Geometry: final body of the model. Coordinates: model frame, mm. A direction names the side the tool comes from. Coordinates: 2 decimals unless noted, no trailing zeros. Loops run counter-clockwise (first coordinate to the right, second up) from the corner with the lowest first, then second, coordinate; pieces in that order, holes last. Notation, with made-up numbers: (53, 41) - (59, 41) arc R13 ccw to (59, 59) - close; hole circle Ø7 at (-5, 17). An arc over 180 degrees is marked (long way). Return JSON: item names as keys, results as strings.
from build123d import *

# Parameters (mm, degrees)
SKETCH1_R           = 1
BOSS_EXTRUDE1_DEPTH = 4
SKETCH2_R           = 1
CUT_EXTRUDE1_DEPTH  = 4


with BuildPart() as part:
    # Sketch1 → Boss-Extrude1 (new body)
    with BuildSketch(Plane(origin=(0, 0, 0), x_dir=(1, 0, 0), z_dir=(0, 1, 0))):
        Polygon((0, 0), (47.5, 0), (72.5, 25), (72.5, 50), (62.5, 50), (62.5, 29.142135624), (43.357864376, 10), (0, 10), (-43.357864376, 10), (-62.5, 29.142135624), (-62.5, 50), (-72.5, 50), (-72.5, 25), (-47.5, 0), align=None)
        with Locations(Location((10, 5, 0), (0, 0, 270))):
            Circle(SKETCH1_R, mode=Mode.SUBTRACT)
        with Locations(Location((0, 5, 0), (0, 0, 270))):
            Circle(SKETCH1_R, mode=Mode.SUBTRACT)
        with Locations(Location((-10, 5, 0), (0, 0, 90))):
            Circle(SKETCH1_R, mode=Mode.SUBTRACT)
    extrude(amount=BOSS_EXTRUDE1_DEPTH)

    # Sketch2 → Cut-Extrude1 (cut)
    with BuildSketch(Plane(origin=(0, 4, 0), x_dir=(1, 0, 0), z_dir=(0, 1, 0))):
        with Locations(Location((67.5, 47.5, 0), (0, 0, 270))):
            Circle(SKETCH2_R)
        with Locations(Location((67.5, 43.5, 0), (0, 0, 270))):
            Circle(SKETCH2_R)
        with Locations(Location((-67.5, 43.5, 0), (0, 0, 90))):
            Circle(SKETCH2_R)
        with Locations(Location((-67.5, 47.5, 0), (0, 0, 90))):
            Circle(SKETCH2_R)
    extrude(amount=-CUT_EXTRUDE1_DEPTH, mode=Mode.SUBTRACT)


solid = part.part
Item 1: Section query B-B, the plane z = -31. Return loops of the section in (x, y).
Worked out:
{"outline": "(-72.5, 0) - (-62.5, 0) - (-62.5, 4) - (-72.5, 4) - close; (62.5, 0) - (72.5, 0) - (72.5, 4) - (62.5, 4) - close"}
Item 2: Section query D-D, the plane z = -21. Return loops of the section in (x, y).
Worked out:
{"outline": "(-68.5, 0) - (-54.36, 0) - (-54.36, 4) - (-68.5, 4) - close; (54.36, 0) - (68.5, 0) - (68.5, 4) - (54.36, 4) - close"}
Item 3: First-contact query: pin 1 Ø1.6 at (x, z) = (-10, -5) entering from +Y. Flat tip, straight axial feed; report the tip coordinate or a pass-through.
Worked out:
{"pin 1": "through"}
Item 4: Reachability of faces 1 (the face through (53.063, 1.972, -19.705)), 2 (the face through (59.8, 2, -12.3)) from +Z, -Z, +X, -X, +Y, -Y: full face, straight path, thin tool, end or side. Return the list, or none.
Worked out:
{"face 1": "-Z, +Y, -Y", "face 2": "+Z, +X, +Y, -Y"}
Item 5: Section query A-A, the plane y = 3.2. Return loops of the section in (x, z).
Worked out:
{"outline": "(-72.5, -50) - (-62.5, -50) - (-62.5, -29.14) - (-43.36, -10) - (43.36, -10) - (62.5, -29.14) - (62.5, -50) - (72.5, -50) - (72.5, -25) - (47.5, 0) - (-47.5, 0) - (-72.5, -25) - close; hole circle Ø2 at (-67.5, -47.5); hole circle Ø2 at (-67.5, -43.5); hole circle Ø2 at (-10, -5); hole circle Ø2 at (0, -5); hole circle Ø2 at (10, -5); hole circle Ø2 at (67.5, -47.5); hole circle Ø2 at (67.5, -43.5)"}
Item 6: Mould query, pull axis X, two halves, no side actions, for faces 3 (the face through (-62.5, 2, -39)), 4 (the face through (68, 2, -50)), 5 (the face through (1, 2, -10)), 6 (the face through (72.5, 2, -37)). Classes: +X half, -X half, draft (parallel to the pull), parting line (faces both ways), or undercut.
Worked out:
{"face 3": "undercut", "face 4": "draft", "face 5": "undercut", "face 6": "+X half"}
Item 7: Section query C-C, the plane x = -29.5. Return loops of the section in (y, z).
Worked out:
{"outline": "(0, -10) - (4, -10) - (4, 0) - (0, 0) - close"}
Item 8: Ray query, probe 1 along X at (y, z) = (2, -43.5); probe 2 along Z at (x, y) = (67.5, 2.65); probe 3 along X at (y, z) = (1.95, -42). Return the intervals inside material, ascending. Write a range as from..to.
Worked out:
{"probe 1": "-72.5..-68.5, -66.5..-62.5, 62.5..66.5, 68.5..72.5", "probe 2": "-50..-48.5, -46.5..-44.5, -42.5..-20", "probe 3": "-72.5..-62.5, 62.5..72.5"}
